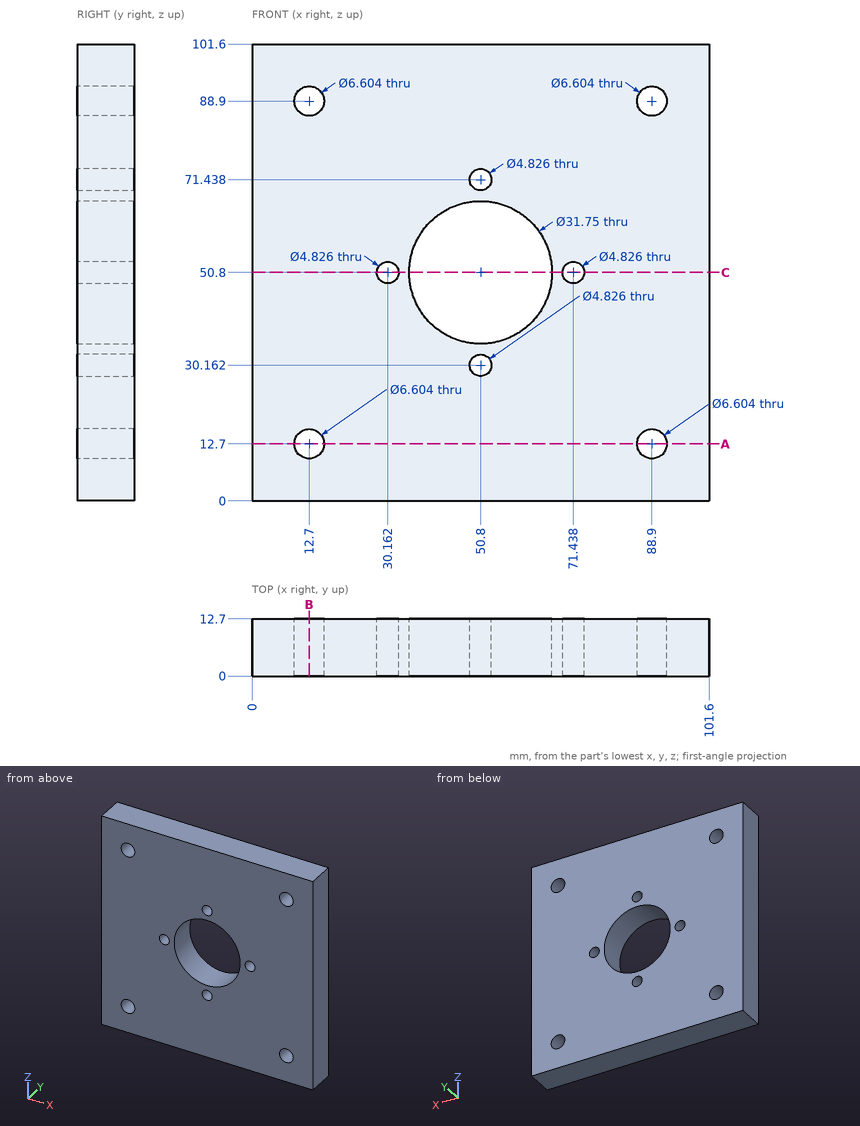
Geometry: see drawing. Coordinates: mm, zero at the bounding-box minimum. Round coordinates to 2 decimals unless told otherwise and drop trailing zeros. Order: outer loops, then holes, each group sorted by start corner. A loop starts at its lowest first (then second) coordinate and runs counter-clockwise, first axis right, second up. Notation, with made-up numbers: (-23, 76) - (15, 76) arc R16 ccw to (15, 105) - close; hole circle Ø1 at (54, -31). An arc over 180 degrees is marked (long way). One line per question, with ' | ' between items. Start each with the question number.
1) Cut plane C-C, the plane z = 50.8. Give the number of separate pieces and of enclosed holes in the cut face.
2) Cut plane A-A, the plane z = 12.7. Return the cut outline in (x, y), then the cut area to 3 significant figures.
3) Cut plane B-B, the plane x = 12.7. Return the cut outline in (y, z).
4) Ray query, probe 1 along X at (y, z) = (8.5, 88.9); probe 2 along X at (y, z) = (2.75, 30); probe 3 along X at (y, z) = (3.5, 15). Return the intervals inside material, ascending.
5) Contact query for a flat-ended pin moving along its axis: P1, Ø6, axis at x = 12.7, z = 12.7, coming from the +Y side. Output: stop coordinate, or through.
Worked out:
1) separate pieces: 4 | enclosed holes: 0
2) outline: (0, 0) - (9.4, 0) - (9.4, 12.7) - (0, 12.7) - close; (16, 0) - (85.6, 0) - (85.6, 12.7) - (16, 12.7) - close; (92.2, 0) - (101.6, 0) - (101.6, 12.7) - (92.2, 12.7) - close | area: 1,120 mm^2
3) outline: (0, 0) - (12.7, 0) - (12.7, 9.4) - (0, 9.4) - close; (0, 16) - (12.7, 16) - (12.7, 85.6) - (0, 85.6) - close; (0, 92.2) - (12.7, 92.2) - (12.7, 101.6) - (0, 101.6) - close
4) probe 1: x = 0 to 9.4, 16 to 85.6, 92.2 to 101.6 | probe 2: x = 0 to 48.39, 53.21 to 101.6 | probe 3: x = 0 to 10.33, 15.07 to 86.53, 91.27 to 101.6
5) P1: passes through
